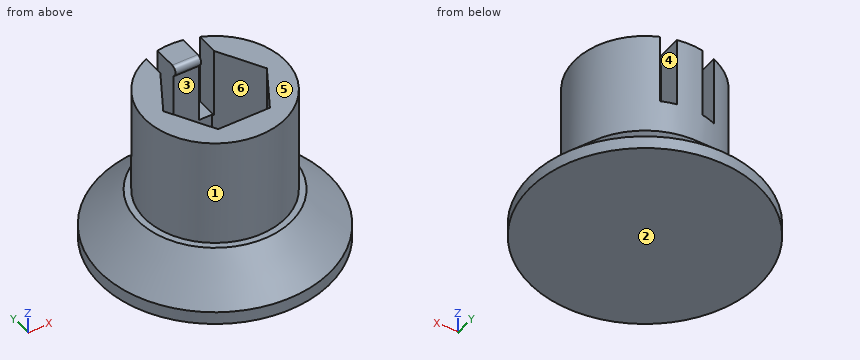
```python
from build123d import *

# Parameters (mm, degrees)
SKETCH_R          = 9
PAD_DEPTH         = 4
SKETCH001_R       = 5.5
PAD001_DEPTH      = 8.5
POCKET_DEPTH      = 9
SKETCH003_W       = 1.1
SKETCH003_H       = 4.61522
POCKET001_DEPTH   = 5.5
PAD002_DEPTH      = 1
PAD002_DEPTH_BACK = 1
FILLET_R          = 0.4
CHAMFER_SIZE      = 3


with BuildPart() as part:
    # Sketch (on XY_Plane of Origin) → Pad (new body)
    with BuildSketch(Plane.XY):
        Circle(SKETCH_R)
    extrude(amount=PAD_DEPTH)

    # Sketch001 (on Face3 of Pad) → Pad001 (join)
    with BuildSketch(Plane.XY.offset(4)):
        Circle(SKETCH001_R)
    extrude(amount=PAD001_DEPTH)

    # Sketch002 (on Face5 of Pad001) → Pocket (cut)
    with BuildSketch(Plane.XY.offset(12.5)):
        Polygon((2.020726, 3.5), (-2.020726, 3.5), (-4.041452, 0), (-2.020726, -3.5), (2.020726, -3.5), (4.041452, 0), align=None)
    extrude(amount=-POCKET_DEPTH, mode=Mode.SUBTRACT)

    # Sketch003 (on Face5 of Pocket) → Pocket001 (cut)
    with BuildSketch(Plane.XY.offset(12.5)):
        with Locations((-1.55, 4.391028)):
            Rectangle(SKETCH003_W, SKETCH003_H)
    pocket001 = extrude(amount=-POCKET001_DEPTH, mode=Mode.SUBTRACT)

    # Mirrored: Pocket001 across Sketch003 V_Axis
    add(pocket001.mirror(Plane(origin=(0, 0, 12.5), x_dir=(0, 0, 1), z_dir=(1, 0, 0))), mode=Mode.SUBTRACT)

    # Sketch004 (on YZ_Plane of Origin) → Pad002 (join, two sides)
    with BuildSketch(Plane.YZ) as pad002_sk:
        Polygon((3.6, 12.5), (3.6, 11.5), (2.8, 12.5), align=None)
    extrude(amount=PAD002_DEPTH)
    extrude(pad002_sk.sketch, amount=-PAD002_DEPTH_BACK)

    # Fillet
    fillet_edges = [part.edges().sort_by_distance(p)[0] for p in [
        (0, 2.8, 12.5),
    ]]
    fillet(fillet_edges, radius=FILLET_R)

    # Chamfer
    chamfer_edges = [part.edges().sort_by_distance(p)[0] for p in [
        (-9, 0, 4),
    ]]
    chamfer(chamfer_edges, length=CHAMFER_SIZE)


solid = part.part
```
Part model, mm, in its own coordinate system. Face numbers are marked on the shaded views. A direction names the side the tool comes from. Coordinates: 2 decimals unless noted, no trailing zeros. Order: outer loops, then holes, each group sorted by start corner. A loop starts at its lowest first (then second) coordinate and runs counter-clockwise, first axis right, second up. Notation, with made-up numbers: (34.25, 41) - (60.25, 41) arc R27 cw to (60.25, 59) - close; hole circle Ø3 at (-30.75, 52.25). An arc over 180 degrees is marked (long way). Return JSON: item names as keys, results as strings. Group by question number.
Item 1: Drill centre lines: probe 1 along Y at (x, z) = (-0.25, 6.5); probe 2 along Z at (x, y) = (0.25, 2.25); probe 3 along X at (y, z) = (1, 8.25). Where is each one in solid material? Low to high. Write a range as from..to.
Item 2: Pull direction Y, two halves, no side cores. Call the marked faces 1, 2 and 3: pulls with the +Y half, pulls with the -Y half, needs draft (parallel to the pull), parting line crosses it, or undercut.
Item 3: Pin check, flat tips, straight feed: pin 1 (1.1 mm diameter, centred on y = 4, z = 9.5, fed in from +X); pin 2 (3 mm diameter, centred on x = 5.5, y = -6, fed in from +Z); pin 3 (2 mm diameter, centred on x = 0.5, z = 6.5, fed in from -Y). Stop position of each tip, or through.
Item 4: Cut at C-C (z = 1.75). List the corners of the cut face in (x, y).
Item 5: Cut at B-B (x = 0). List the corners of the cut face in (y, z) (3 decimals), plus the area to 3 significant figures.
Item 6: Which spindle directions (+Z, -Z, +X, -X, +Y, -Y) get a long thin tool onto all of the face, cutting with end or side? Do the marked faces 4, 5 and 6. Say none if no direction does.
Item 7: Cut at A-A (z = 7.5). List the corners of the cut face in (x, y).
Check values:
{
 "1": {"probe 1": "y = -5.49..-3.5, 3.5..5.49", "probe 2": "z = 0..3.5", "probe 3": "x = -5.41..-3.46, 3.46..5.41"},
 "2": {"face 1": "parting line crosses it", "face 2": "needs draft", "face 3": "undercut"},
 "3": {"pin 1": "stops at x = 4.28", "pin 2": "stops at z = 3.36", "pin 3": "stops at y = -5.5"},
 "4": {"outline": "circle Ø16.5 at (0, 0)"},
 "5": {"outline": "(-9, 0) - (9, 0) - (9, 1) - (6, 4) - (5.5, 4) - (5.5, 12.5) - (3.632, 12.5) arc R0.4 ccw to (3.32, 11.85) - (3.5, 11.625) - (3.5, 3.5) - (-3.5, 3.5) - (-3.5, 12.5) - (-5.5, 12.5) - (-5.5, 4) - (-6, 4) - (-9, 1) - close", "area": "93.7 mm2"},
 "6": {"face 4": "+Z, +Y", "face 5": "+Z, +X, -X, +Y, -Y", "face 6": "+Z"},
 "7": {"outline": "(-4.04, 0) - (-2.1, 3.36) - (-2.1, 5.08) arc R5.5 ccw (long way) to (2.1, 5.08) - (2.1, 3.36) - (4.04, 0) - (2.02, -3.5) - (-2.02, -3.5) - close; (-1, 3.5) - (1, 3.5) - (1, 5.41) arc R5.5 ccw to (-1, 5.41) - close"}
}
